The listing builds one solid part. Answer for the finished solid, in the listing's coordinates (mm). A direction names the side the tool comes from. Give positions to 0.01 mm unless a question says otherwise; leave off trailing zeros. Write each loop counter-clockwise with the first axis right and the second up, starting at its lowest first coordinate (ties: lowest second). Pieces come first, ordered by that corner, then holes.
Autodesk Inventor part; units mm, degrees
ref_plane "YZ Plane" through (0, 0, 0) normal (1, 0, 0) x (0, 1, 0)
ref_plane "XZ Plane" through (0, 0, 0) normal (0, 1, 0) x (-1, 0, 0)
ref_plane "XY Plane" through (0, 0, 0) normal (0, 0, 1) x (1, 0, 0)
sketch "Sketch1" plane through (0, 0, 0) normal (0, 0, 1) x (1, 0, 0)
  line L0 (0, 0) -> (6.35, 0)
  line L1 (6.35, 0) -> (6.35, 10.16)
  line L2 (0, 17.78) -> (1.5875, 17.78)
  line L3 (1.5875, 17.78) -> (5.7488, 12.0191)
  arc A0 (6.35, 10.16) -> (5.7488, 12.0191) centre (3.175, 10.16) ccw
  line L4 (0, 0) -> (3.175, 0)
  line L5 (1.5875, 17.78) -> (1.5875, 0)
  line L6 (6.35, 0) -> (1.5875, 0)
  line L7 (0, -3.556) -> (0, 21.336)
  dimension "d0" = 6.35
  dimension "d3" = 1.5875
  dimension "d4" = 3.175
  dimension "d9" = 10.16
  dimension "d10" = 17.78
revolve "Revolution1" add sketch "Sketch1" angle 360 about axis through (0, -10, 0) along (0, 1, 0) contours L5 L3 A0 L1 L0
sketch "Sketch2" plane through (0, 0, 0) normal (0, -1, 0) x (1, 0, 0)
  circle A0 centre (0, 0) radius 1.5875
  circle A1 centre (0, 0) radius 1.5875
  circle A2 centre (0, 0) radius 5.3975
  dimension "d6" = 10.795
extrude "Extrusion1" add sketch "Sketch2" along normal blind 5.08
properties part number "tipthick1024"
Item 1: Which of the six approach directions +Z, -Z, +X, -X, +Y, -Y give full straight-line access (tool end or side, diameter ignored) to faces 4 (the face through (-3.978, -2.504, -3.648)), 5 (the face through (-1.3, -5.08, 1.3))?
Conclusion:
face 4: -Y
face 5: +Z, -Z, +X, -X, -Y
Item 2: Consider probe 1 along Z at (x, y) = (0, 10.25); probe 2 along Z at (x, y) = (-0.5, 8.5). Determine where each line is inside the solid, lowest interval first.
Conclusion:
probe 1: z = -6.35 to -1.59, 1.59 to 6.35
probe 2: z = -6.33 to -1.51, 1.51 to 6.33
Item 3: A cutting plane is placed at A-A, the plane y = 13.5. Give the vertices of the cut face in (x, z) (1 decimal), plus the area to 3 significant figures.
Conclusion:
outline: circle Ø9.4 at (0, 0); hole circle Ø3.2 at (0, 0)
area: 60.9 mm2
Item 4: Determine the mould class of faces 1 (the face through (-1.38, 5.15, 6.2)), 2 (the face through (-3, 0, 5)), 3 (the face through (-0.34, 6.19, -1.55)) for opening direction Z: pulls with the +Z half, pulls with the -Z half, needs draft (parallel to the pull), parting line crosses it, or undercut.
Conclusion:
face 1: parting line crosses it
face 2: needs draft
face 3: undercut
Item 5: Each of these flat-tipped pins is pushed along its axis until it touches: P1, Ø4, axis at x = 5, y = 5.5, coming from the -Z side; P2, Ø5, axis at x = -2.5, y = 14.5, coming from the -Z side; P3, Ø5, axis at y = 9.5, z = -4, coming from the -X side. Where does it stop, or does it pass through?
Conclusion:
P1: stops at z = -5.6
P2: stops at z = -5.41
P3: stops at x = -6.17
